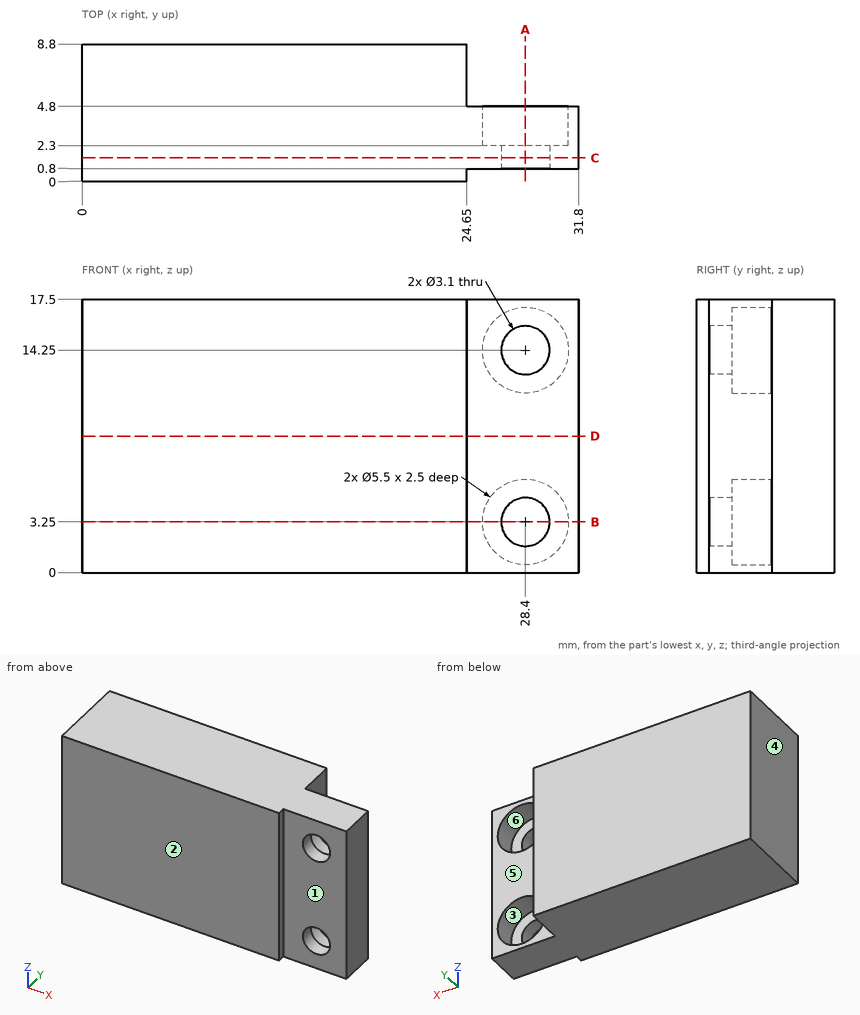
Job drawing, mm, ordinate dimensions from the low corner. One solid piece. A direction names the side the tool comes from. Round coordinates to 2 decimals unless told otherwise and drop trailing zeros. Order: outer loops, then holes, each group sorted by start corner. A loop starts at its lowest first (then second) coordinate and runs counter-clockwise, first axis right, second up. Notation, with made-up numbers: M 2.5,47 L 6.5,47 A19 cw 6.5,72 Z; hole C 27,-12.75 d8. An arc over 180 degrees is marked long. Write each question's results on one line, items separated by ' | '. Start each with the question number.
(1) Probe probe 1 along Z at (x, y) = (28.4, 3.1); probe 2 along Z at (x, y) = (28.4, 1.7); probe 3 along X at (y, z) = (1.25, 14.25). List the from-to ranges inside material, lowest first. Write a range as from..to.
(2) Saw through at B-B, the plane z = 3.25. Give the cut face in (x, y), then the cut area to 3 significant figures.
(3) Saw through at C-C, the plane y = 1.5. Give the cut face in (x, z), then the cut area to 3 significant figures.
(4) Two-plate mould, pull along X, no slides. Class the marked faces 3, 4, 5 and 6: pulls with the +X half, pulls with the -X half, needs draft (parallel to the pull), parting line crosses it, or undercut.
(5) Saw through at D-D, the plane z = 8.75. Give the cut face in (x, y).
(6) Drop flat-ended pins along their axis: pin 1 (1.2 mm diameter, centred on y = 7, z = 7, fed in from +X); pin 2 (7 mm diameter, centred on x = 28.4, z = 14.25, fed in from -Y); pin 3 (2.5 mm diameter, centred on x = 28.4, z = 14.25, fed in from +Y); pin 4 (5.5 mm diameter, centred on x = 28, z = 10, fed in from +Y). Give the stop position or say it passes through.
(7) Which spindle directions (+Z, -Z, +X, -X, +Y, -Y) get a long thin tool onto all of the face, cutting with end or side? Do the marked faces 1 and 2. Say none if no direction does.
(8) Saw through at A-A, the plane x = 28.4. Give the cut face in (y, z), then the cut area to 3 significant figures.
Established:
1) probe 1: z = 0..0.5, 6..11.5, 17..17.5 | probe 2: z = 0..1.7, 4.8..12.7, 15.8..17.5 | probe 3: x = 0..26.85, 29.95..31.8
2) outline: M 0,0 L 24.65,0 L 24.65,0.8 L 26.85,0.8 L 26.85,2.3 L 25.65,2.3 L 25.65,4.8 L 24.65,4.8 L 24.65,8.8 L 0,8.8 Z; M 29.95,0.8 L 31.8,0.8 L 31.8,4.8 L 31.15,4.8 L 31.15,2.3 L 29.95,2.3 Z | area: 227 mm^2
3) outline: M 0,0 L 31.8,0 L 31.8,17.5 L 0,17.5 Z; hole C 28.4,3.25 d3.1; hole C 28.4,14.25 d3.1 | area: 541 mm^2
4) face 3: undercut | face 4: pulls with the -X half | face 5: needs draft | face 6: undercut
5) outline: M 0,0 L 24.65,0 L 24.65,0.8 L 31.8,0.8 L 31.8,4.8 L 24.65,4.8 L 24.65,8.8 L 0,8.8 Z
6) pin 1: stops at x = 24.65 | pin 2: stops at y = 0.8 | pin 3: passes through | pin 4: stops at y = 4.8
7) face 1: +Z, -Z, +X, -Y | face 2: +Z, -Z, +X, -X, -Y
8) outline: M 0.8,0 L 4.8,0 L 4.8,0.5 L 2.3,0.5 L 2.3,1.7 L 0.8,1.7 Z; M 0.8,4.8 L 2.3,4.8 L 2.3,6 L 4.8,6 L 4.8,11.5 L 2.3,11.5 L 2.3,12.7 L 0.8,12.7 Z; M 0.8,15.8 L 2.3,15.8 L 2.3,17 L 4.8,17 L 4.8,17.5 L 0.8,17.5 Z | area: 33.2 mm^2
